Verification items for this drawing (mm, ordinates from the low corner). A direction names the side the tool comes from. Round coordinates to 2 decimals unless told otherwise and drop trailing zeros. Loops run counter-clockwise (first coordinate to the right, second up) from the corner with the lowest first, then second, coordinate; pieces in that order, holes last. Notation, with made-up numbers: M -19.5,-33.75 L 28.5,-33.75 A27 ccw 28.5,0.25 Z; hole C -14.5,46.25 d10. An arc over 180 degrees is marked long. Write item = value, one per line. Start each with the question number.
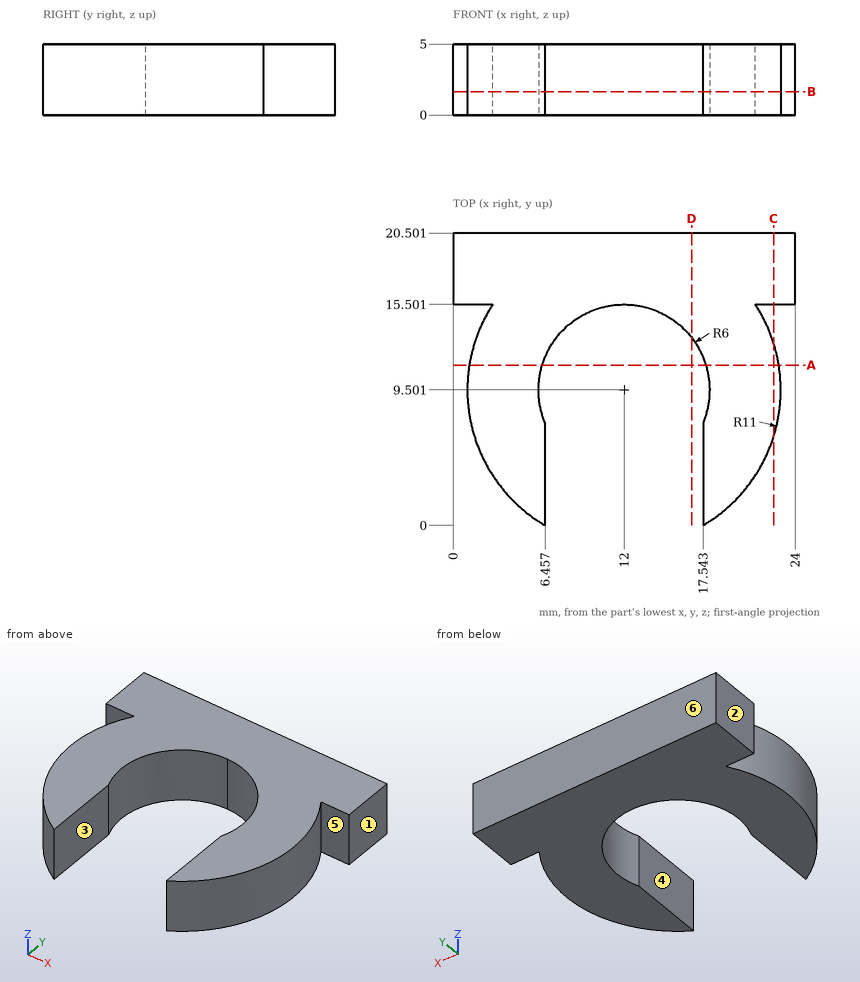
1. Gauge pin test, flat ends, axial feed: P1, Ø1.5, axis at y = 3.5, z = 2.5, coming from the -X side (1 decimal); P2, Ø2.5, axis at y = 2, z = 1.5, coming from the +X side; P3, Ø3, axis at x = 1, z = 2, coming from the -Y side (1 decimal). Record the tip position at first contact, or that the pin passes through.
2. Section check D-D, the plane x = 16.75. Enter the section's corners in (y, z), and give its area (3 significant figures).
3. Section check C-C, the plane x = 22.5. Enter the section's corners in (y, z), and give its area (3 significant figures).
4. Section check A-A, the plane y = 11.25. Enter the section's corners in (x, z).
5. Tool access check on the marked faces 5 and 6. Record the directions out of +Z, -Z, +X, -X, +Y, -Y that give a thin tool (end or side, any length) a straight path to the whole face; none if there is none.
6. Mould release check, pull along X, two halves, no side actions. Record for the marked faces 1, 2, 3 and 4: pulls with the +X half, pulls with the -X half, needs draft (parallel to the pull), parting line crosses it, or undercut.
7. Thickness scan on line 1 (X direction, y = 5.75, z = 1.45); line 2 (Y direction, x = 2.5, z = 3) (1 decimal); line 3 (X direction, y = 3.25, z = 4.4). Record the ranges inside material, lowest first.
8. Section check B-B, the plane z = 1.65. Enter the section's corners in (x, y) (1 decimal), and give its area (3 significant figures).
Computed values:
q1.P1 = 2.3
q1.P2 = 21.05
q1.P3 = 4
q2.outline = M 13.17,0 L 20.5,0 L 20.5,5 L 13.17,5 Z
q2.area = 36.7 mm2
q3.outline = M 6.22,0 L 12.78,0 L 12.78,5 L 6.22,5 Z; M 15.5,0 L 20.5,0 L 20.5,5 L 15.5,5 Z
q3.area = 57.8 mm2
q4.outline = M 1.14,0 L 6.26,0 L 6.26,5 L 1.14,5 Z; M 17.74,0 L 22.86,0 L 22.86,5 L 17.74,5 Z
q5.face_5 = +Z, -Z, +X
q5.face_6 = +Z, -Z, +X, -X, +Y
q6.face_1 = pulls with the +X half
q6.face_2 = pulls with the -X half
q6.face_3 = undercut
q6.face_4 = undercut
q7.line_1 = 1.66 to 6.46, 17.54 to 22.34
q7.line_2 = 4 to 15, 15.5 to 20.5
q7.line_3 = 2.95 to 6.46, 17.54 to 21.05
q8.outline = M 0,15.5 L 2.8,15.5 A11 ccw 6.5,0 L 6.5,7.2 A6 cw long 17.5,7.2 L 17.5,0 A11 ccw 21.2,15.5 L 24,15.5 L 24,20.5 L 0,20.5 Z
q8.area = 261 mm2
